Autodesk Inventor part; units mm, degrees
ref_plane "YZ Plane" through (0, 0, 0) normal (1, 0, 0) x (0, 1, 0)
ref_plane "XZ Plane" through (0, 0, 0) normal (0, 1, 0) x (-1, 0, 0)
ref_plane "XY Plane" through (0, 0, 0) normal (0, 0, 1) x (1, 0, 0)
sketch "Sketch1" plane through (0, 0, 0) normal (0, 0, 1) x (1, 0, 0)
  line L0 (-107.2757, 7.2736) -> (3.8493, 7.2736)
  line L1 (3.8493, 7.2736) -> (3.8493, -30.8264)
  line L2 (3.8493, -30.8264) -> (-107.2757, -30.8264)
  line L3 (-107.2757, -30.8264) -> (-107.2757, 7.2736)
  circle A0 centre (-72.1471, 0.8391) radius 1.5875
  circle A1 centre (-53.9997, -24.4192) radius 1.5875
  circle A2 centre (-3.5671, 0.8391) radius 1.5875
  circle A3 centre (-66.6357, -18.1264) radius 8.89
  circle A4 centre (-42.8867, -18.1264) radius 8.89
  circle A5 centre (-81.8757, -19.3964) radius 6.35
  circle A6 centre (-11.1367, -19.3964) radius 6.35
  line L4 (-42.8867, -30.8264) -> (-4.7867, -30.8264)
  line L5 (-4.7867, -30.8264) -> (-4.7867, -28.2864)
  line L6 (-4.7867, -28.2864) -> (-42.8867, -28.2864)
  line L7 (-42.8867, -28.2864) -> (-42.8867, -30.8264)
  line L8 (-46.3681, 7.2736) -> (-20.9681, 7.2736)
  point P0 (0, 0)
  dimension "d2" = 111.125
  dimension "d3" = 38.1
  dimension "d4" = 3.175
  dimension "d5" = 3.175
  dimension "d6" = 3.175
  dimension "d7" = 12.7
  dimension "d8" = 12.7
  dimension "d9" = 17.78
  dimension "d10" = 17.78
  dimension "d11" = 12.7
  dimension "d12" = 12.7
  dimension "d13" = 23.749
  dimension "d14" = 11.43
  dimension "d15" = 11.43
  dimension "d16" = 15.24
  dimension "d17" = 31.75
  dimension "d18" = 6.4345
  dimension "d19" = 6.4345
  dimension "d20" = 68.58
  dimension "d21" = 6.4071
  dimension "d22" = 11.1131
  dimension "d23" = 5.5114
  dimension "d24" = 2.54
  dimension "d25" = 38.1
  dimension "d26" = 0
  dimension "d27" = 25.4
extrude "Extrusion1" add sketch "Sketch1" along normal blind 3.175 contours L0 L1 L2 L5 L6 L7 L3
properties part number "Dish_Injector_Wall"
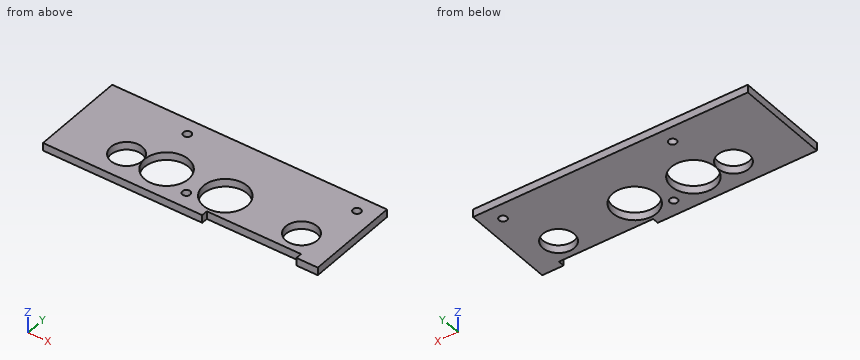
Build history of the part. All positions in model axes, mm. Coordinates: 2 decimals unless noted, no trailing zeros. Write each loop counter-clockwise with the first axis right and the second up, starting at its lowest first coordinate (ties: lowest second). Pieces come first, ordered by that corner, then holes.
(1) Pin check, flat tip, straight feed: pin 1 Ø2.5 at (x, y) = (-3.57, 0.84) entering from -Z. Stop position of the tip, or through.
(2) Cut at B-B on z = 0.7. State how many separate pieces and enclosed holes the cut face has, and give its area (3 significant figures).
(3) Drill centre lines: line 1 (Y direction, x = -67, z = 2.05); line 2 (X direction, y = -20, z = 2.65); line 3 (Y direction, x = -72.5, z = 2.1). Where is each one in solid material? Low to high.
(4) Cut at C-C on y = -16.5. List the corners of the cut face in (x, z) (3 decimals).
(5) Cut at D-D on x = -82. List the corners of the cut face in (y, z) (3 decimals), and give its area (3 significant figures).
(6) Cut at A-A on x = -50.5. List the corners of the cut face in (y, z) (3 decimals).
Working result:
1. pin 1: passes through
2. separate pieces: 1
2. enclosed holes: 7
2. area: 3,360 mm2
3. line 1: y = -30.83 to -27.01, -9.24 to 7.27
3. line 2: x = -107.28 to -88.2, -75.55 to -75.33, -57.95 to -51.58, -34.2 to -17.46, -4.82 to 3.85
3. line 3: y = -30.83 to -24.81, -11.44 to -0.71, 2.39 to 7.27
4. outline: (-107.276, 0) - (-87.527, 0) - (-87.527, 3.175) - (-107.276, 3.175) - close; (-76.225, 0) - (-75.376, 0) - (-75.376, 3.175) - (-76.225, 3.175) - close; (-57.896, 0) - (-51.627, 0) - (-51.627, 3.175) - (-57.896, 3.175) - close; (-34.147, 0) - (-16.788, 0) - (-16.788, 3.175) - (-34.147, 3.175) - close; (-5.486, 0) - (3.849, 0) - (3.849, 3.175) - (-5.486, 3.175) - close
5. outline: (-30.826, 0) - (-25.745, 0) - (-25.745, 3.175) - (-30.826, 3.175) - close; (-13.048, 0) - (7.274, 0) - (7.274, 3.175) - (-13.048, 3.175) - close
5. area: 80.7 mm2
6. outline: (-30.826, 0) - (-22.717, 0) - (-22.717, 3.175) - (-30.826, 3.175) - close; (-13.536, 0) - (7.274, 0) - (7.274, 3.175) - (-13.536, 3.175) - close
